from build123d import *

# Parameters (mm, degrees)
BOSS_EXTRUDE1_DEPTH = 20
SKETCH2_R           = 13.5
CUT_EXTRUDE1_DEPTH  = 40
SKETCH4_R           = 1.5
CUT_EXTRUDE2_DEPTH  = 40
SKETCH5_R           = 1.5
CUT_EXTRUDE3_DEPTH  = 40
FILLET1_R           = 10
FILLET2_R           = 5


with BuildPart() as part:
    # Sketch1 → Boss-Extrude1 (new body, symmetric)
    with BuildSketch(Plane.XY):
        Polygon((0, 0), (22, 0), (22, 1.5), (1.5, 1.5), (1.5, 40), (0, 40), align=None)
    extrude(amount=BOSS_EXTRUDE1_DEPTH, both=True)

    # Sketch2 → Cut-Extrude1 (cut)
    with BuildSketch(Plane(origin=(1.5, 0, 0), x_dir=(0, 0, -1), z_dir=(1, 0, 0))):
        with Locations((0, 20)):
            Circle(SKETCH2_R)
    extrude(amount=-CUT_EXTRUDE1_DEPTH, mode=Mode.SUBTRACT)

    # Sketch4 → Cut-Extrude2 (cut)
    with BuildSketch(Plane(origin=(1.5, 0, 0), x_dir=(0, 0, -1), z_dir=(1, 0, 0))):
        with Locations((16.25, 20)):
            Circle(SKETCH4_R)
        with Locations((14.072912811, 11.875)):
            Circle(SKETCH4_R)
        with Locations((8.125, 5.927087189)):
            Circle(SKETCH4_R)
        with Locations((0, 3.75)):
            Circle(SKETCH4_R)
        with Locations((-8.125, 5.927087189)):
            Circle(SKETCH4_R)
        with Locations((-14.072912811, 11.875)):
            Circle(SKETCH4_R)
        with Locations((-16.25, 20)):
            Circle(SKETCH4_R)
        with Locations((-14.072912811, 28.125)):
            Circle(SKETCH4_R)
        with Locations((-8.125, 34.072912811)):
            Circle(SKETCH4_R)
        with Locations((0, 36.25)):
            Circle(SKETCH4_R)
        with Locations((8.125, 34.072912811)):
            Circle(SKETCH4_R)
        with Locations((14.072912811, 28.125)):
            Circle(SKETCH4_R)
    extrude(amount=-CUT_EXTRUDE2_DEPTH, mode=Mode.SUBTRACT)

    # Sketch5 → Cut-Extrude3 (cut)
    with BuildSketch(Plane(origin=(0, 1.5, 0), x_dir=(1, 0, 0), z_dir=(0, 1, 0))):
        with Locations((5, 15)):
            Circle(SKETCH5_R)
        with Locations((11, 15)):
            Circle(SKETCH5_R)
        with Locations((17, 15)):
            Circle(SKETCH5_R)
        with Locations((17, -15)):
            Circle(SKETCH5_R)
        with Locations((11, -15)):
            Circle(SKETCH5_R)
        with Locations((5, -15)):
            Circle(SKETCH5_R)
    extrude(amount=-CUT_EXTRUDE3_DEPTH, mode=Mode.SUBTRACT)

    # Fillet1
    fillet1_edges = [part.edges().sort_by_distance(p)[0] for p in [
        (0.75, 40, 20),
        (0.75, 40, -20),
    ]]
    fillet(fillet1_edges, radius=FILLET1_R)

    # Fillet2
    fillet2_edges = [part.edges().sort_by_distance(p)[0] for p in [
        (22, 0.75, 20),
        (22, 0.75, -20),
    ]]
    fillet(fillet2_edges, radius=FILLET2_R)


solid = part.part
Here's how the part is built. I have some questions about the finished solid (model axes, mm). A direction names the side the tool comes from. Round coordinates to 2 decimals unless told otherwise and drop trailing zeros. Order: outer loops, then holes, each group sorted by start corner. A loop starts at its lowest first (then second) coordinate and runs counter-clockwise, first axis right, second up. Notation, with made-up numbers: (70.25, 16.25) -> (98.25, 16.25) arc R31 cw to (98.25, 47.25) -> close; hole circle Ø1 at (-2.5, 61.5). An arc over 180 degrees is marked (long way). Return JSON: item names as keys, results as strings.
Q1. For pin 1 Ø5 at (y, z) = (20, 16.25) entering from +X; pin 2 Ø1.5 at (y, z) = (10, -7) entering from -X; pin 3 Ø10 at (x, z) = (16.5, -7.5) entering from +Y, each with a flat end and sliding along its axis, tell me the tip position at first contact or that it passes through.
Filled sheet:
{"pin 1": "stops at x = 1.5", "pin 2": "passes through", "pin 3": "stops at y = 1.5"}
Q2. Which directions (+Z, -Z, +X, -X, +Y, -Y) give clear straight access to the entire face, cutting with the end or side of a thin tool? Please do faces 4 (the flat face through (12, 1.5, 0)), 5 (the cylindrical face through (0.76, 21.01, -15.14)).
Filled sheet:
{"face 4": "+Z, -Z, +X, +Y", "face 5": "+X, -X"}
Q3. If we section it at D-D on y = 21: List the corners of the cut face in (x, z) for me, plus the area to 3 significant figures.
Filled sheet:
{"outline": "(0, -20) -> (1.5, -20) -> (1.5, -17.37) -> (0, -17.37) -> close; (0, -15.13) -> (1.5, -15.13) -> (1.5, -13.46) -> (0, -13.46) -> close; (0, 13.46) -> (1.5, 13.46) -> (1.5, 15.13) -> (0, 15.13) -> close; (0, 17.37) -> (1.5, 17.37) -> (1.5, 20) -> (0, 20) -> close", "area": "12.9 mm^2"}
Q4. If we mould it in two halves opening along Z, with no side actions, what happens to faces 1 (the flat face through (11, 0, 0)), 2 (the cylindrical face through (0.74, 36.99, 17.15)), 3 (the cylindrical face through (0.76, 35.09, 9.23))? For each: released by +Z, released by -Z, zero draft, split by the parting line, or undercut.
Filled sheet:
{"face 1": "zero draft", "face 2": "released by +Z", "face 3": "undercut"}
Q5. If we section it at A-A on y = 3.75: List the corners of the cut face in (x, z) for me.
Filled sheet:
{"outline": "(0, -20) -> (1.5, -20) -> (1.5, -1.5) -> (0, -1.5) -> close; (0, 1.5) -> (1.5, 1.5) -> (1.5, 20) -> (0, 20) -> close"}
Q6. If we section it at B-B on z = 0: List the corners of the cut face in (x, y) for me, plus the area to 4 significant figures.
Filled sheet:
{"outline": "(0, 0) -> (22, 0) -> (22, 1.5) -> (1.5, 1.5) -> (1.5, 2.25) -> (0, 2.25) -> close; (0, 5.25) -> (1.5, 5.25) -> (1.5, 6.5) -> (0, 6.5) -> close; (0, 33.5) -> (1.5, 33.5) -> (1.5, 34.75) -> (0, 34.75) -> close; (0, 37.75) -> (1.5, 37.75) -> (1.5, 40) -> (0, 40) -> close", "area": "41.25 mm^2"}
Q7. I need wall thicknesses on line 1 along Z through (x, y) = (5, 1.25); line 2 along X through (y, z) = (0.4, 15); line 3 along Y through (x, z) = (21.25, 12.5). Which ranges of each line are inside material? Lowest first, please. Write a range as from..to.
Filled sheet:
{"line 1": "z = -20..-16.5, -13.5..13.5, 16.5..20", "line 2": "x = 0..3.5, 6.5..9.5, 12.5..15.5, 18.5..22", "line 3": "y = 0..1.5"}
Q8. If we section it at C-C on x = 11: List the corners of the cut face in (y, z) for me, plus the area to 3 significant figures.
Filled sheet:
{"outline": "(0, -20) -> (1.5, -20) -> (1.5, -16.5) -> (0, -16.5) -> close; (0, -13.5) -> (1.5, -13.5) -> (1.5, 13.5) -> (0, 13.5) -> close; (0, 16.5) -> (1.5, 16.5) -> (1.5, 20) -> (0, 20) -> close", "area": "51.0 mm^2"}
